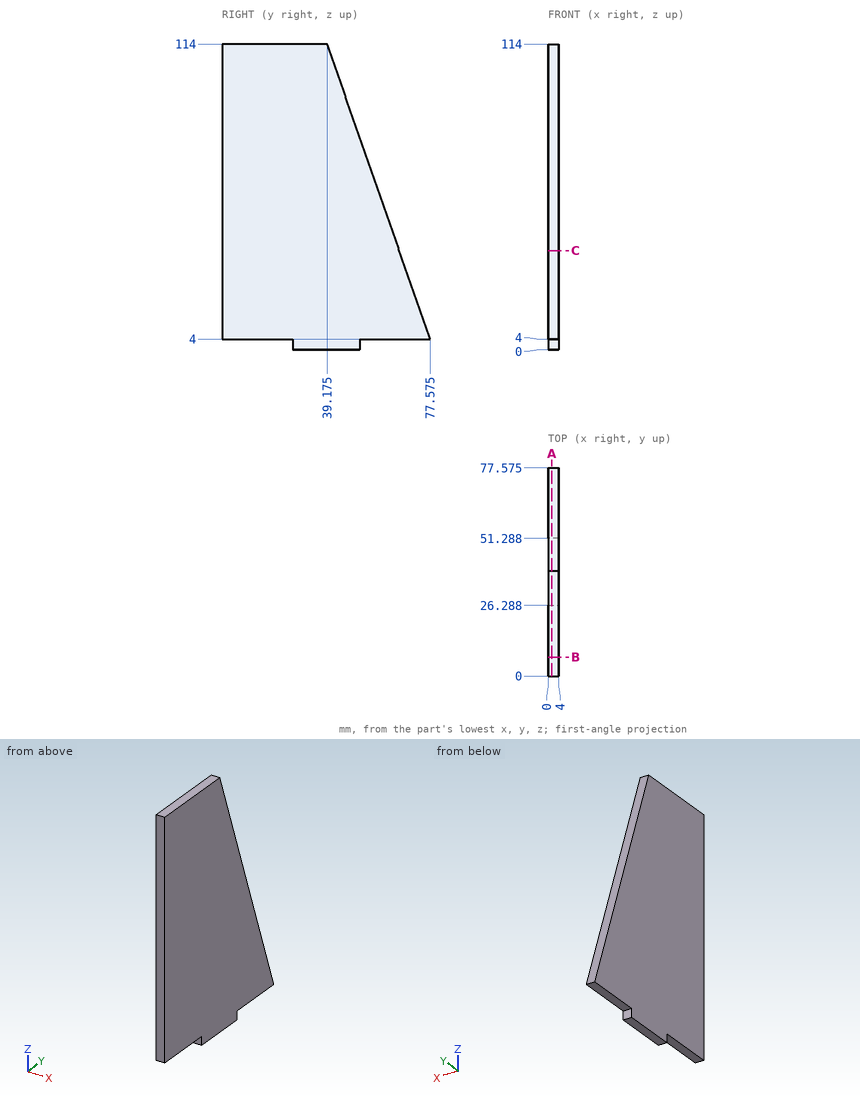
Geometry: see drawing. Coordinates: mm, zero at the bounding-box minimum. Round coordinates to 2 decimals unless told otherwise and drop trailing zeros. Write each loop counter-clockwise with the first axis right and the second up, starting at its lowest first coordinate (ties: lowest second). Pieces come first, ordered by that corner, then holes. Notation, with made-up numbers: M -37,32 L -29,32 A21 cw -29,37 Z; hole C 45.25,73.5 d7. An arc over 180 degrees is marked long. Answer as a JSON object with one key per item and string values. Group by question number.
(1) Ray query, line 1 (Y direction, x = 1.95, z = 41); line 2 (Y direction, x = 0.45, z = 55). Return the intervals inside material, ascending. Write a range as [from, to].
(2) Section query C-C on z = 37. Output: boundary loops of the cut face in (x, y) (1 decimal).
(3) First-contact query: pin 1 (2 mm diameter, centred on x = 2, z = 2.5, fed in from -Y); pin 2 (1 mm diameter, centred on x = 1, z = 31, fed in from +Y) (1 decimal); pin 3 (1 mm diameter, centred on x = 2.5, z = 34, fed in from +Y); pin 4 (2 mm diameter, centred on y = 17, z = 33, fed in from -X). Flat tips, straight axial feed; report the tip coordinate or a pass-through.
(4) Section query B-B on y = 7. Output: boundary loops of the cut face in (x, z).
(5) Section query A-A on x = 1.35. Output: boundary loops of the cut face in (y, z) (1 decimal), then the cut area to 3 significant figures.
Computed values:
{
 "1": {"line 1": "[0, 64.66]", "line 2": "[0, 59.77]"},
 "2": {"outline": "M 0,0 L 4,0 L 4,66.1 L 0,66.1 Z"},
 "3": {"pin 1": "y = 26.29", "pin 2": "y = 68.3", "pin 3": "y = 67.28", "pin 4": "x = 0"},
 "4": {"outline": "M 0,4 L 4,4 L 4,114 L 0,114 Z"},
 "5": {"outline": "M 0,4 L 26.3,4 L 26.3,0 L 51.3,0 L 51.3,4 L 77.6,4 L 39.2,114 L 0,114 Z", "area": "6,520 mm^2"}
}
